```python
from build123d import *

# Parameters (mm, degrees)
BASEHEAD_DEPTH = 5.969


with BuildPart() as part:
    # Sketch1 → BaseHead (new body)
    with BuildSketch(Plane(origin=(0, 0, 0), x_dir=(0, 0, -1), z_dir=(1, 0, 0))):
        Polygon((6.35, 3.666174209), (6.35, -3.666174209), (0, -7.332348419), (-6.35, -3.666174209), (-6.35, 3.666174209), (0, 7.332348419), align=None)
    extrude(amount=BASEHEAD_DEPTH)

    # BodySke → BaseBody (revolve)
    with BuildSketch(Plane.XY):
        Polygon((0, 0), (56.769, 0), (56.769, 3.12928), (55.92953, 3.96875), (0, 3.96875), align=None)
    revolve(axis=Axis((0, 0, 0), (1, 0, 0)))

    # Sketch3 → HeadChamfer (revolve, cut)
    with BuildSketch(Plane.XY):
        Polygon((0, 6.35), (4.233333333, 13.682348419), (4.233333333, 20.032348419), (-12.7, 20.032348419), (-12.7, 6.35), align=None)
    revolve(axis=Axis((0, 0, 0), (1, 0, 0)), mode=Mode.SUBTRACT)


solid = part.part
```
Source: CAD feature listing. Evaluate the final solid. Frame: model axes, mm. A direction names the side the tool comes from. Coordinates: 2 decimals unless noted, no trailing zeros. Loops run counter-clockwise (first coordinate to the right, second up) from the corner with the lowest first, then second, coordinate; pieces in that order, holes last. Notation, with made-up numbers: M -19.5,71 L 13.5,71 A26 cw 13.5,97 Z; hole C 42,20 d5. An arc over 180 degrees is marked long. Use a Markdown table: item, result. Add a question column.
Q1. Access query for faces 1 (the cylindrical face through (30.6, -0.86, -3.874)), 2 (the flat face through (3, 0, 6.35)). Directions: +Z, -Z, +X, -X, +Y, -Y. A direction counts if a zero-diameter tool reaches every point of the face in a straight line with its end or side. Return the directions, or none.
Q2. Material intervals for L1, parallel to X at y = -2.75, z = -4; L2, parallel to Z at x = 28, y = -1.5, sorted ascending.
Q3. First-contact query: pin 1 (5 mm diameter, centred on x = 14, z = -1, fed in from +Y); pin 2 (3 mm diameter, centred on x = 46.5, z = -3.5, fed in from -Y); pin 3 (6 mm diameter, centred on y = -5.5, z = -3.5, fed in from +X). Flat tips, straight axial feed; report the tip coordinate or a pass-through.
Q4. Section query A-A, the plane x = 35. Return loops of the section in (y, z).
Result:
| question | item | result |
|---|---|---|
| 1 | face 1 | +X |
| 1 | face 2 | +Z, +X, -X, +Y, -Y |
| 2 | L1 | x = 0 to 5.97 |
| 2 | L2 | z = -3.67 to 3.67 |
| 3 | pin 1 | stops at y = 3.97 |
| 3 | pin 2 | stops at y = -3.43 |
| 3 | pin 3 | stops at x = 56.38 |
| 4 | outline | C 0,0 d7.94 |
